Build history of the part. All positions in model axes, mm. A direction names the side the tool comes from. Coordinates: 2 decimals unless noted, no trailing zeros. Write each loop counter-clockwise with the first axis right and the second up, starting at its lowest first coordinate (ties: lowest second). Pieces come first, ordered by that corner, then holes. Notation, with made-up numbers: (6.25, 83.5) -> (16.25, 83.5) arc R28 ccw to (16.25, 121.5) -> close; hole circle Ø5 at (52, 10). An arc over 180 degrees is marked (long way). Write each question's results on one line, items separated by ' | '. Start each with the question number.
Q1. Saw through at D-D on y = -3.5. Give the cut face in (x, z).
Q2. Drill centre lines: line 1 (X direction, y = -2.75, z = 2.75); line 2 (X direction, y = -5.5, z = 24.5); line 3 (X direction, y = 5.25, z = 5.75). Where is each one in solid material? Low to high.
Q3. Saw through at C-C on x = -3.75. Give the cut face in (y, z), and give its area (3 significant figures).
Q4. Drop flat-ended pins along their axis: pin 1 Ø2 at (x, z) = (-6, 16) entering from +Y; pin 2 Ø5.5 at (x, z) = (4.5, 15.5) entering from -Y; pin 3 Ø1.5 at (x, z) = (-4, 7) entering from -Y. Give the stop position or say it passes through.
Q5. Two-plate mould, pull along Y, no slides. Class faces 1 (the face through (8.179, 2.576, 13.064)), 2 (the face through (-4.571, 0.648, 13.064)), 3 (the face through (0, -4, 0)): released by +Y, released by -Y, zero draft, split by the parting line, or undercut.
Q6. Saw through at B-B on y = 1.5. Give the cut face in (x, z), and give its area (3 significant figures).
Q7. Tool access for faces 4 (the face through (4.63, 0.69, 13.06)), 5 (the face through (0, -4, 26.5)): list every direction of +Z, -Z, +X, -X, +Y, -Y with a clear straight run to the whole face (end or side of a thin tool).
from build123d import *

# Parameters (mm, degrees)
F0_R     = 8.575
F1_DEPTH = 26.5
F3_DEPTH = 26.5


with BuildPart() as f1:
    # F0 (on Top) → F1 (new body)
    with BuildSketch(Plane.XY):
        Circle(F0_R)
    extrude(amount=F1_DEPTH)

    # F2 (on face) → F3 (cut)
    with BuildSketch(Plane(origin=(0, 0, 0), x_dir=(1, 0, 0), z_dir=(0, 0, -1))):
        Polygon((0, 2.6737620788), (-4.114496766, 5.6631189606), (-2.542898848, 0.8262379212), align=None)
        Polygon((-1.571597918, -2.1631189606), (-2.542898848, 0.8262379212), (-6.6573956141, -2.1631189606), align=None)
        Polygon((1.571597918, -2.1631189606), (-1.571597918, -2.1631189606), (0, -7), align=None)
        Polygon((6.6573956141, -2.1631189606), (2.542898848, 0.8262379212), (1.571597918, -2.1631189606), align=None)
        Polygon((4.114496766, 5.6631189606), (0, 2.6737620788), (2.542898848, 0.8262379212), align=None)
        Polygon((0, 2.6737620788), (-2.542898848, 0.8262379212), (-1.571597918, -2.1631189606), (1.571597918, -2.1631189606), (2.542898848, 0.8262379212), align=None)
    extrude(amount=-F3_DEPTH, mode=Mode.SUBTRACT)


solid = f1.part
Returned:
1) outline: (-7.83, 0) -> (-3.41, 0) -> (-3.41, 26.5) -> (-7.83, 26.5) -> close; (-1.14, 0) -> (1.14, 0) -> (1.14, 26.5) -> (-1.14, 26.5) -> close; (3.41, 0) -> (7.83, 0) -> (7.83, 26.5) -> (3.41, 26.5) -> close
2) line 1: x = -8.12 to -3.17, -0.1 to 0.1, 3.17 to 8.12 | line 2: x = -6.58 to -4.06, -3.89 to 3.89, 4.06 to 6.58 | line 3: x = -6.78 to -0.57, 0.57 to 6.78
3) outline: (-7.71, 0) -> (-5.4, 0) -> (-5.4, 26.5) -> (-7.71, 26.5) -> close; (-4.54, 0) -> (0.05, 0) -> (0.05, 26.5) -> (-4.54, 26.5) -> close; (2.16, 0) -> (7.71, 0) -> (7.71, 26.5) -> (2.16, 26.5) -> close | area: 330 mm2
4) pin 1: stops at y = 6.97 | pin 2: stops at y = -8.39 | pin 3: stops at y = -7.94
5) face 1: split by the parting line | face 2: undercut | face 3: zero draft
6) outline: (-8.44, 0) -> (-5.74, 0) -> (-5.74, 26.5) -> (-8.44, 26.5) -> close; (5.74, 0) -> (8.44, 0) -> (8.44, 26.5) -> (5.74, 26.5) -> close | area: 143 mm2
7) face 4: +Z, -Z | face 5: +Z, +X, -X, +Y, -Y
